Verification items for the finished model (mm, model axes). Face numbers are marked on the shaded views. Give positions to 0.01 mm unless a question says otherwise; leave off trailing zeros. Loops run counter-clockwise (first coordinate to the right, second up) from the corner with the lowest first, then second, coordinate; pieces in that order, holes last. Notation, with made-up numbers: (6, 68.5) - (55, 68.5) arc R28 ccw to (55, 89.5) - close; hole circle Ø5 at (-1, 68.5). An arc over 180 degrees is marked (long way). Use one line per item in the form item = value.
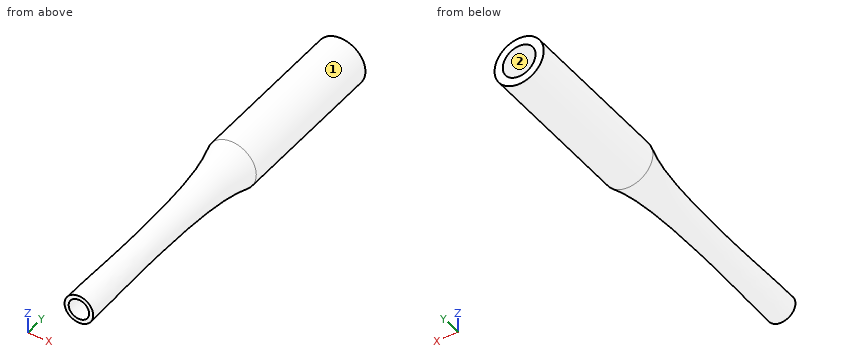
```python
from build123d import *

# Parameters (mm, degrees)
F2_R     = 7.9375
F3_DEPTH = 304.801
F4_R     = 12.7
F5_DEPTH = 57.15
F6_R     = 11.90625
F7_DEPTH = 76.2


with BuildPart() as f1:
    # F0 (on Right) → F1 (revolve)
    with BuildSketch(Plane.YZ):
        with BuildLine():
            add(Edge.make_bspline(
                [(-304.8, 11.1125), (-285.75, 11.1125), (-242.2367029758, 9.5359179721), (-161.7897503824, 10.6315785702), (-135.382, 16.51), (-127, 19.05)],
                knots=[0, 0, 0, 0, 0.3497446097, 0.7455097749, 1, 1, 1, 1], degree=3))
            Line((-304.8, 11.1125), (-304.8, 0))
            Line((-304.8, 0), (0, 0))
            Line((0, 0), (0, 19.05))
            Line((0, 19.05), (-127, 19.05))
        make_face()
    revolve(axis=Axis((0, -152.4, 0), (0, 1, 0)))

    # F2 (on face) → F3 (cut, through all)
    with BuildSketch(Plane.XZ.offset(304.8)):
        Circle(F2_R)
    extrude(amount=-F3_DEPTH, mode=Mode.SUBTRACT)

    # F4 (on face) → F5 (cut)
    with BuildSketch(Plane(origin=(0, 0, 0), x_dir=(-1, 0, 0), z_dir=(0, 1, 0))):
        Circle(F4_R)
    extrude(amount=-F5_DEPTH, mode=Mode.SUBTRACT)

    # F6 (on face) → F7 (cut)
    with BuildSketch(Plane(origin=(0, -57.15, 0), x_dir=(-1, 0, 0), z_dir=(0, 1, 0))):
        Circle(F6_R)
    extrude(amount=-F7_DEPTH, mode=Mode.SUBTRACT)


solid = f1.part
```
1. Section check A-A, the plane y = -49.5. Record the cut outline in (x, z), then the cut area to 3 significant figures.
Result set:
outline = circle Ø38.1 at (0, 0); hole circle Ø25.4 at (0, 0)
area = 633 mm²
2. Scan lines: probe 1 along X at (y, z) = (-80.5, 0.5); probe 2 along Z at (x, y) = (5, -61); probe 3 along X at (y, z) = (-171, 2). Record each from-to range of solid material in increasing order.
Result set:
probe_1 = -19.04 to -11.9, 11.9 to 19.04
probe_2 = -18.38 to -10.81, 10.81 to 18.38
probe_3 = -11.57 to -7.68, 7.68 to 11.57
3. Depth check by flat-ended pin: pin 1 Ø12.5 at (x, z) = (-4.5, -1.5) entering from +Y; pin 2 Ø7 at (x, z) = (2.5, 1) entering from +Y; pin 3 Ø1 at (x, y) = (-9, -138) entering from -Z; pin 4 Ø2 at (y, z) = (-39, 0) entering from -X. Enter the tip coordinate at first touch or a pass-through.
Result set:
pin_1 = -133.35
pin_2 = through
pin_3 = -13.79
pin_4 = -19.05
4. Draft check along Z on the marked faces 1 and 2. Enter one of: released by +Z, released by -Z, zero draft, split by the parting line, or undercut.
Result set:
face_1 = split by the parting line
face_2 = undercut
